The listing builds one solid part. Answer for the finished solid, in the listing's coordinates (mm). A direction names the side the tool comes from. Round coordinates to 2 decimals unless told otherwise and drop trailing zeros. Loops run counter-clockwise (first coordinate to the right, second up) from the corner with the lowest first, then second, coordinate; pieces in that order, holes last. Notation, with made-up numbers: (13, 80) - (35, 80) arc R28 ccw to (35, 118) - close; hole circle Ø9 at (82, 89). An arc over 180 degrees is marked (long way). One line per item, written item: value.
```python
from build123d import *

# Parameters (mm, degrees)
BOSS_EXTRUDE1_DEPTH = 19.05
SKETCH2_R           = 3.3782
CUT_EXTRUDE1_DEPTH  = 43.081104502
FILLET1_R           = 3.175


with BuildPart() as part:
    # Sketch1 → Boss-Extrude1 (new body)
    with BuildSketch(Plane.XY):
        with BuildLine():
            Line((-15.875, 0), (-33.998547486, 0))
            Line((-33.998547486, 0), (-33.998547486, -6.35))
            Line((-33.998547486, -6.35), (-21.298547486, -6.35))
            ThreePointArc((-21.298547486, -6.35), (0, -22.225), (21.298547486, -6.35))
            Line((21.298547486, -6.35), (33.998547486, -6.35))
            Line((33.998547486, -6.35), (33.998547486, 0))
            Line((33.998547486, 0), (15.875, 0))
            ThreePointArc((15.875, 0), (0, -15.875), (-15.875, 0))
        make_face()
    extrude(amount=BOSS_EXTRUDE1_DEPTH)

    # Sketch2 → Cut-Extrude1 (cut, through all)
    with BuildSketch(Plane.XZ.offset(6.35)):
        with Locations(Location((27.648547486, 9.525, 0), (0, 0, 270))):
            Circle(SKETCH2_R)
        with Locations(Location((-27.648547486, 9.525, 0), (0, 0, 270))):
            Circle(SKETCH2_R)
    extrude(amount=-CUT_EXTRUDE1_DEPTH, mode=Mode.SUBTRACT)

    # Fillet1
    fillet1_edges = [part.edges().sort_by_distance(p)[0] for p in [
        (15.875, 0, 9.525),
        (-15.875, 0, 9.525),
    ]]
    fillet(fillet1_edges, radius=FILLET1_R)


solid = part.part
```
1) A cutting plane is placed at B-B on z = 10.75. Give the vertices of the cut face in (x, y) (3 decimals).
Final values:
outline: (-33.999, -6.35) - (-30.797, -6.35) - (-30.797, 0) - (-33.999, 0) - close; (-24.5, -6.35) - (-21.299, -6.35) arc R22.225 ccw to (21.299, -6.35) - (24.5, -6.35) - (24.5, 0) - (18.784, 0) arc R3.175 ccw to (15.653, -2.646) arc R15.875 cw to (-15.653, -2.646) arc R3.175 ccw to (-18.784, 0) - (-24.5, 0) - close; (30.797, -6.35) - (33.999, -6.35) - (33.999, 0) - (30.797, 0) - close
2) For a pull along Z with two mould halves and no side action, classify faces 1 (the cylindrical face through (-30.646, -3.219, 7.966)), 2 (the flat face through (-3, -16, 0)), 3 (the flat face through (25, 0, 12)) as released by +Z, released by -Z, zero draft, split by the parting line, or undercut.
Final values:
face 1: undercut
face 2: released by -Z
face 3: zero draft
3) Each of these flat-tipped pins is pushed along its axis until it touches: pin 1 Ø5 at (y, z) = (-9.5, 8) entering from -X; pin 2 Ø3 at (y, z) = (-17, 6.5) entering from +X; pin 3 Ø10 at (x, z) = (28, 5.5) entering from -Y. Where does it stop, or does it pass through?
Final values:
pin 1: x = -21.09
pin 2: x = 15.93
pin 3: y = -6.35
4) Consider L1, parallel to Y at x = -30, z = 18; L2, parallel to X at y = -10, z = 14.25; L3, parallel to X at y = -9.5, z = 2. Determine where each line is inside the solid, lowest interval first.
Final values:
L1: -6.35 to 0
L2: -19.85 to -12.33, 12.33 to 19.85
L3: -20.09 to -12.72, 12.72 to 20.09
5) A cutting plane is placed at D-D on y = -3.5. Give the vertices of the cut face in (x, z) (3 decimals), and give its area (3 significant figures).
Final values:
outline: (-33.999, 0) - (-15.484, 0) - (-15.484, 19.05) - (-33.999, 19.05) - close; (15.484, 0) - (33.999, 0) - (33.999, 19.05) - (15.484, 19.05) - close; hole circle Ø6.756 at (-27.649, 9.525); hole circle Ø6.756 at (27.649, 9.525)
area: 634 mm2
6) For faces 4 (the flat face through (-31, -6.35, 7)), 5 (the cylindrical face through (16.71, -0.77, 9.66)), 6 (the flat face through (25, -6.35, 7)), determine the directions among +Z, -Z, +X, -X, +Y, -Y from which every point of the face is accessible in a straight line to the end or side of a thin tool.
Final values:
face 4: +Z, -Z, -X, -Y
face 5: +Z, -Z, +Y
face 6: +Z, -Z, +X, -Y
7) A cutting plane is placed at A-A on y = -7.25. Give the vertices of the cut face in (x, z), and give its area (3 significant figures).
Final values:
outline: (-21.01, 0) - (-14.12, 0) - (-14.12, 19.05) - (-21.01, 19.05) - close; (14.12, 0) - (21.01, 0) - (21.01, 19.05) - (14.12, 19.05) - close
area: 262 mm2
8) A cutting plane is placed at C-C on x = 27. Give the vertices of the cut face in (y, z).
Final values:
outline: (-6.35, 0) - (0, 0) - (0, 6.21) - (-6.35, 6.21) - close; (-6.35, 12.84) - (0, 12.84) - (0, 19.05) - (-6.35, 19.05) - close
